from build123d import *

# Parameters (mm, degrees)
BOSS_EXTRUDE1_DEPTH = 50.8
SKETCH3_R           = 2.4892
CUT_EXTRUDE1_DEPTH  = 4.175
SKETCH4_R           = 2.4892
CUT_EXTRUDE2_DEPTH  = 4.175


with BuildPart() as part:
    # Sketch1 → Boss-Extrude1 (new body)
    with BuildSketch(Plane(origin=(0, 0, 0), x_dir=(1, 0, 0), z_dir=(0, 1, 0))):
        Polygon((3.175, 3.175), (25.4, 3.175), (25.4, 0), (0, 0), (0, 25.4), (3.175, 25.4), align=None)
    extrude(amount=BOSS_EXTRUDE1_DEPTH)

    # Sketch3 → Cut-Extrude1 (cut, through all)
    with BuildSketch(Plane(origin=(0, 0, -3.175), x_dir=(-1, 0, 0), z_dir=(0, 0, -1))):
        with Locations((-14.2875, 25.4)):
            Circle(SKETCH3_R)
    extrude(amount=-CUT_EXTRUDE1_DEPTH, mode=Mode.SUBTRACT)

    # Sketch4 → Cut-Extrude2 (cut, through all)
    with BuildSketch(Plane(origin=(3.175, 0, 0), x_dir=(0, 0, -1), z_dir=(1, 0, 0))):
        with Locations((14.2875, 12.7)):
            Circle(SKETCH4_R)
        with Locations((14.2875, 38.1)):
            Circle(SKETCH4_R)
    extrude(amount=-CUT_EXTRUDE2_DEPTH, mode=Mode.SUBTRACT)


solid = part.part
Here's how the part is built. I have some questions about the finished solid (model axes, mm). A direction names the side the tool comes from. Give positions to 0.01 mm unless a question says otherwise; leave off trailing zeros. Write each loop counter-clockwise with the first axis right and the second up, starting at its lowest first coordinate (ties: lowest second). Pieces come first, ordered by that corner, then holes. Notation, with made-up numbers: (-6.5, 84) -> (16.5, 84) arc R5 ccw to (16.5, 92) -> close; hole circle Ø4 at (60.5, 57.5). An arc over 180 degrees is marked (long way). Use one line per item in the form item = value. Start each with the question number.
1. Imagine slicing it at B-B on x = 13.75. List the corners of the cut face in (y, z) for me (3 decimals).
2. Thinking about a two-plate mould opening in Y: for faces 1 (the face through (2, 25, -25.4)), 2 (the face through (1.61, 15.168, -13.963)), 3 (the face through (1.61, 35.67, -13.75)), 4 (the face through (7, 50.8, -2)), which applies, +Y half, -Y half, draft (parallel to the pull), parting line (faces both ways), or undercut?
3. On a 3-axis mill with a long thin cutter (end or side, diameter ignored), from which of +Z, -Z, +X, -X, +Y, -Y can I reach the whole of each face in a straight line? I mean faces 5 (the face through (3.175, 25, -14)), 6 (the face through (14.61, 27.87, -1.61)). Say none if no direction works.
4. Imagine slicing it at D-D on x = 6. List the corners of the cut face in (y, z) for me (3 decimals).
5. If I drill on L1, parallel to X at y = 13, z = -7.5 (3 decimals); L2, parallel to Z at x = 4, y = 20 (3 decimals), over which ranges is the centre line in solid material (lowest first)?
6. Imagine slicing it at C-C on z = -7.75. List the corners of the cut face in (x, y) for me (3 decimals), plus the area to 3 significant figures.
7. Will these pins go through, and if not, where does the flat tip stop? pin 1 Ø4.5 at (y, z) = (38.1, -14.29) entering from -X; pin 2 Ø1.5 at (y, z) = (18.5, -6.5) entering from +X (3 decimals).
8. Imagine slicing it at A-A on y = 38.1. List the corners of the cut face in (x, z) for me (3 decimals).
Entries:
q1.outline = (0, -3.175) -> (22.97, -3.175) -> (22.97, 0) -> (0, 0) -> close; (27.83, -3.175) -> (50.8, -3.175) -> (50.8, 0) -> (27.83, 0) -> close
q2.face_1 = draft
q2.face_2 = undercut
q2.face_3 = undercut
q2.face_4 = +Y half
q3.face_5 = -Z, +X, +Y, -Y
q3.face_6 = +Z, -Z
q4.outline = (0, -3.175) -> (50.8, -3.175) -> (50.8, 0) -> (0, 0) -> close
q5.L1 = 0 to 3.175
q5.L2 = -3.175 to 0
q6.outline = (0, 0) -> (3.175, 0) -> (3.175, 50.8) -> (0, 50.8) -> close
q6.area = 161 mm²
q7.pin_1 = through
q7.pin_2 = 3.175
q8.outline = (0, -25.4) -> (3.175, -25.4) -> (3.175, -16.777) -> (0, -16.777) -> close; (0, -11.798) -> (3.175, -11.798) -> (3.175, -3.175) -> (25.4, -3.175) -> (25.4, 0) -> (0, 0) -> close
